```python
from build123d import *

# Parameters (mm, degrees)
SKETCH1_R           = 97.5
BOSS_EXTRUDE1_DEPTH = 650
SKETCH2_R           = 97.5
SKETCH2_R_2         = 67.5
CUT_EXTRUDE4_DEPTH  = 250
SKETCH4_R           = 67.5
CUT_EXTRUDE3_DEPTH  = 98.5
FILLET1_R           = 40
SKETCH5_R           = 67.5
CUT_EXTRUDE5_DEPTH  = 350


with BuildPart() as part:
    # Sketch1 → Boss-Extrude1 (new body)
    with BuildSketch(Plane(origin=(0, 0, 0), x_dir=(1, 0, 0), z_dir=(0, 1, 0))):
        Circle(SKETCH1_R)
    extrude(amount=BOSS_EXTRUDE1_DEPTH)

    # Sketch2 → Cut-Extrude4 (cut)
    with BuildSketch(Plane.XZ):
        Circle(SKETCH2_R)
        Circle(SKETCH2_R_2, mode=Mode.SUBTRACT)
    extrude(amount=-CUT_EXTRUDE4_DEPTH, mode=Mode.SUBTRACT)

    # Sketch4 → Cut-Extrude3 (cut, through all)
    with BuildSketch(Plane.XY):
        with Locations((0, 450)):
            Circle(SKETCH4_R)
    extrude(amount=-CUT_EXTRUDE3_DEPTH, mode=Mode.SUBTRACT)

    # Fillet1
    fillet1_edges = [part.edges().sort_by_distance(p)[0] for p in [
        (-97.5, 650, 0),
    ]]
    fillet(fillet1_edges, radius=FILLET1_R)

    # Sketch5 → Cut-Extrude5 (cut)
    with BuildSketch(Plane.XZ):
        Circle(SKETCH5_R)
    extrude(amount=-CUT_EXTRUDE5_DEPTH, mode=Mode.SUBTRACT)


solid = part.part
```
CAD build for the part. Positions are in the model's coordinates, mm. A direction names the side the tool comes from. Give positions to 0.01 mm unless a question says otherwise; leave off trailing zeros. Loops run counter-clockwise (first coordinate to the right, second up) from the corner with the lowest first, then second, coordinate; pieces in that order, holes last. Notation, with made-up numbers: (-26.75, 20) -> (15.25, 20) arc R14 cw to (15.25, 39) -> close; hole circle Ø7 at (77, 30). An arc over 180 degrees is marked (long way). Use a Markdown table: item, result.
1. Slice it at B-B (y = 309). List the corners of the cut face in (x, z), plus the area to 3 significant figures.
Check result:
| item | result |
|---|---|
| outline | circle Ø195 at (0, 0); hole circle Ø135 at (0, 0) |
| area | 15,600 mm^2 |
2. Mould opens along Y. For faces 1 (the cylindrical face through (-53.57, 299.3, -41.07)), 2 (the flat face through (-1, 350, 1)), 3 (the flat face through (-1, 451, 0)) say: pulls with the +Y half, pulls with the -Y half, needs draft (parallel to the pull), parting line crosses it, or undercut.
Check result:
| item | result |
|---|---|
| face 1 | needs draft |
| face 2 | pulls with the -Y half |
| face 3 | undercut |
3. Flat gauge pins, fed straight in: pin 1 (6 mm diameter, centred on x = 64.5, z = -40, fed in from +Y); pin 2 (3 mm diameter, centred on x = 4, y = 369.5, fed in from -Z); pin 3 (2 mm diameter, centred on x = -39.5, y = 301.5, fed in from -Z). Where does each tip first touch, or does it go through?
Check result:
| item | result |
|---|---|
| pin 1 | stops at y = 646.92 |
| pin 2 | stops at z = -97.47 |
| pin 3 | stops at z = -89.58 |
4. Slice it at D-D (y = 450). List the corners of the cut face in (x, z).
Check result:
| item | result |
|---|---|
| outline | (-67.5, -70.36) -> (-67.5, 0) -> (67.5, 0) -> (67.5, -70.36) arc R97.5 ccw (long way) to start |
5. Wall check: L1, parallel to Z at x = 0, y = 273; L2, parallel to Y at x = 0, z = -50.5; L3, parallel to Y at x = -34, z = 28.5. Give the ranges that are in metal, low to high. Write a range as [from, to].
Check result:
| item | result |
|---|---|
| L1 | z = [-97.5, -67.5], [67.5, 97.5] |
| L2 | y = [350, 382.5], [517.5, 650] |
| L3 | y = [350, 650] |
6. Which spindle directions (+Z, -Z, +X, -X, +Y, -Y) get a long thin tool onto all of the face, cutting with end or side? Do faces 4 (the flat face through (-1, 650, -1)), 5 (the cylindrical face through (-53.57, 408.93, -48.07)). Say none if no direction does.
Check result:
| item | result |
|---|---|
| face 4 | +Z, -Z, +X, -X, +Y |
| face 5 | -Z |
7. Slice it at A-A (x = 0). List the corners of the cut face in (y, z).
Check result:
| item | result |
|---|---|
| outline | (250, -97.5) -> (382.5, -97.5) -> (382.5, 0) -> (517.5, 0) -> (517.5, -97.5) -> (610, -97.5) arc R40 ccw to (650, -57.5) -> (650, 57.5) arc R40 ccw to (610, 97.5) -> (250, 97.5) -> (250, 67.5) -> (350, 67.5) -> (350, -67.5) -> (250, -67.5) -> close |
8. Slice it at C-C (y = 622.5). List the corners of the cut face in (x, z).
Check result:
| item | result |
|---|---|
| outline | circle Ø190.99 at (0, 0) |
